from build123d import *

# Parameters (mm, degrees)
BOSS_EXTRUDE1_START = 0.5
SKETCH1_R           = 40
BOSS_EXTRUDE1_DEPTH = 4
CUT_EXTRUDE1_START  = -6
SKETCH2_R           = 3.025
CUT_EXTRUDE1_DEPTH  = 6
SKETCH3_R           = 5.1
CUT_EXTRUDE2_DEPTH  = 15


with BuildPart() as part:
    # Sketch1 → Boss-Extrude1 (new body)
    with BuildSketch(Plane.XY.offset(BOSS_EXTRUDE1_START)):
        Circle(SKETCH1_R)
    extrude(amount=BOSS_EXTRUDE1_DEPTH)

    # Sketch2 → Cut-Extrude1 (cut)
    with BuildSketch(Plane.XY.offset(4.5).offset(CUT_EXTRUDE1_START)):
        with Locations((0, 34)):
            Circle(SKETCH2_R)
        with Locations((29.444863729, -17)):
            Circle(SKETCH2_R)
        with Locations((-29.444863729, -17)):
            Circle(SKETCH2_R)
        with BuildLine():
            Line((-8.888194417, 39), (8.888194417, 39))
            ThreePointArc((8.888194417, 39), (0, 40), (-8.888194417, 39))
        make_face()
        with BuildLine():
            Line((38.219087956, -11.802597841), (29.330893539, -27.197402159))
            ThreePointArc((29.330893539, -27.197402159), (34.641016151, -20), (38.219087956, -11.802597841))
        make_face()
        with BuildLine():
            Line((-29.330893539, -27.197402159), (-38.219087956, -11.802597841))
            ThreePointArc((-38.219087956, -11.802597841), (-34.641016151, -20), (-29.330893539, -27.197402159))
        make_face()
    extrude(amount=CUT_EXTRUDE1_DEPTH, mode=Mode.SUBTRACT)

    # Sketch3 → Cut-Extrude2 (cut)
    with BuildSketch(Plane.XY.offset(4.5)):
        Circle(SKETCH3_R)
    extrude(amount=-CUT_EXTRUDE2_DEPTH, mode=Mode.SUBTRACT)


solid = part.part
Geometry check sheet. Reference: the model listing, model coordinates, mm. Round coordinates to 2 decimals unless told otherwise and drop trailing zeros. Loops run counter-clockwise (first coordinate to the right, second up) from the corner with the lowest first, then second, coordinate; pieces in that order, holes last. Notation, with made-up numbers: (66, 65.25) - (81, 65.25) arc R19 cw to (81, 96.25) - close; hole circle Ø8 at (47.25, 33.5). An arc over 180 degrees is marked (long way). One line per question, with ' | ' between items. Start each with the question number.
1. Cross-section at C-C on x = 0. Record the cut outline in (y, z) (3 decimals).
2. Scan lines: line 1 (Y direction, x = 0, z = 3.5) (3 decimals); line 2 (X direction, y = -17, z = 2.8); line 3 (X direction, y = 34, z = 3.1) (3 decimals). Record each from-to range of solid material in increasing order. Write a range as [from, to].
3. Draft check along X on faces 1 (the face through (2.4, -4.5, 2.5)), 2 (the face through (-33.71, -19.61, 2.47)), 3 (the face through (8, 0, 0.5)). Enter one of: released by +X, released by -X, zero draft, split by the parting line, or undercut.
4. Cross-section at A-A on y = 0. Record the cut outline in (x, z).
5. Cross-section at B-B on z = 3.4. Record the cut outline in (x, y) (3 decimals).
6. Cross-section at D-D on y = -17. Record the cut outline in (x, z).
7. Depth check by flat-ended pin: pin 1 (3.5 mm diameter, centred on x = 29.44, y = -17, fed in from -Z); pin 2 (1.5 mm diameter, centred on x = -21, z = 1.5, fed in from +Y); pin 3 (2 mm diameter, centred on y = -5.5, z = 1.5, fed in from -X); pin 4 (1 mm diameter, centred on x = -17, z = 3.5, fed in from +Y). Enter the tip coordinate at first touch or a pass-through.
Taken from the geometry:
1) outline: (-40, 0.5) - (-5.1, 0.5) - (-5.1, 4.5) - (-40, 4.5) - close; (5.1, 0.5) - (30.975, 0.5) - (30.975, 4.5) - (5.1, 4.5) - close; (37.025, 0.5) - (39, 0.5) - (39, 4.5) - (37.025, 4.5) - close
2) line 1: [-40, -5.1], [5.1, 30.975], [37.025, 39] | line 2: [-35.22, -32.47], [-26.42, 26.42], [32.47, 35.22] | line 3: [-21.071, -3.025], [3.025, 21.071]
3) face 1: undercut | face 2: released by -X | face 3: zero draft
4) outline: (-40, 0.5) - (-5.1, 0.5) - (-5.1, 4.5) - (-40, 4.5) - close; (5.1, 0.5) - (40, 0.5) - (40, 4.5) - (5.1, 4.5) - close
5) outline: (-38.219, -11.803) - (-29.331, -27.197) arc R40 ccw to (29.331, -27.197) - (38.219, -11.803) arc R40 ccw to (8.888, 39) - (-8.888, 39) arc R40 ccw to start; hole circle Ø6.05 at (-29.445, -17); hole circle Ø10.2 at (0, 0); hole circle Ø6.05 at (0, 34); hole circle Ø6.05 at (29.445, -17)
6) outline: (-35.22, 0.5) - (-32.47, 0.5) - (-32.47, 4.5) - (-35.22, 4.5) - close; (-26.42, 0.5) - (26.42, 0.5) - (26.42, 4.5) - (-26.42, 4.5) - close; (32.47, 0.5) - (35.22, 0.5) - (35.22, 4.5) - (32.47, 4.5) - close
7) pin 1: through | pin 2: y = 34.5 | pin 3: x = -39.75 | pin 4: y = 36.44
